Could you check a few things on this model? Use its own coordinates, in mm. Face numbers are marked on the shaded views. A direction names the side the tool comes from. Round coordinates to 2 decimals unless told otherwise and drop trailing zeros. Order: outer loops, then holes, each group sorted by start corner. A loop starts at its lowest first (then second) coordinate and runs counter-clockwise, first axis right, second up.
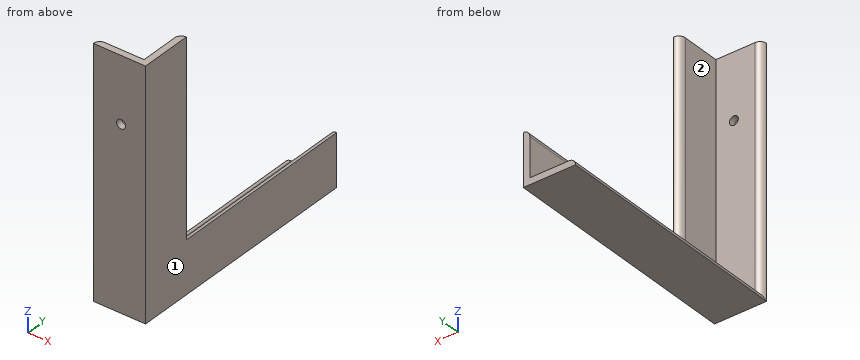
```python
from build123d import *

# Parameters (mm, degrees)
PAD003_DEPTH    = 150
PAD004_DEPTH    = 150
SKETCH012_R     = 2.75
POCKET001_DEPTH = 150.001


with BuildPart() as part:
    # Sketch003 → Pad003 (new body)
    with BuildSketch(Plane.XY):
        with BuildLine():
            Line((0, 32), (0, 0))
            Line((0, 0), (-32, 0))
            ThreePointArc((-28, 4), (-30.828427, 2.828427), (-32, 0))
            Line((-4, 4), (-28, 4))
            Line((-4, 28), (-4, 4))
            ThreePointArc((0, 32), (-2.828427, 30.828427), (-4, 28))
        make_face()
    extrude(amount=PAD003_DEPTH)

    # Sketch004 (on Face3 of Pad003) → Pad004 (new body)
    with BuildSketch(Plane.XZ):
        with BuildLine():
            Line((-32, 0), (0, 0))
            Line((0, 0), (0, 32))
            ThreePointArc((0, 32), (-2.828427, 30.828427), (-4, 28))
            Line((-4, 4), (-4, 28))
            Line((-28, 4), (-4, 4))
            ThreePointArc((-28, 4), (-30.828427, 2.828427), (-32, 0))
        make_face()
    extrude(amount=-PAD004_DEPTH)

    # Sketch012 (on Face9 of Pad004) → Pocket001 (cut, through all)
    with BuildSketch(Plane.XZ):
        with Locations((-15, 110)):
            Circle(SKETCH012_R)
    extrude(amount=-POCKET001_DEPTH, mode=Mode.SUBTRACT)


solid = part.part
```
Q1. For the marked faces 1 and 2, which set-ups out of +Z, -Z, +X, -X, +Y, -Y let a thin tool reach every point of the face, with its end or its side?
Q2. Imagine slicing it at C-C, the plane y = 69.5. Please give me the cut outline in (x, z), then the cut area to 3 significant figures.
Q3. For P1, Ø2, axis at x = -4.5, y = 86.5, coming from the +Z side; P2, Ø7, axis at x = -21.5, z = 76.5, coming from the +Y side; P3, Ø1.5, axis at x = -18.5, y = 111, coming from the +Z side, each with a flat end and sliding along its axis, tell me the tip position at first contact or that it passes through.
Q4. I need wall thicknesses on L1, parallel to Z at x = -15, y = 1.35; L2, parallel to Y at x = -18.5, z = 73. Which ranges of each line are inside material? Lowest first, please.
Q5. Imagine slicing it at B-B, the plane x = -15. Please give me the cut outline in (y, z).
Q6. Imagine slicing it at A-A, the plane z = 110. Please give me the cut outline in (x, y).
Filled in:
1. face 1: +Z, -Z, +X, +Y, -Y
1. face 2: +Z, -X, +Y
2. outline: (-32, 0) - (0, 0) - (0, 32) arc R4 ccw to (-4, 28) - (-4, 4) - (-28, 4) arc R4 ccw to start
2. area: 233 mm2
3. P1: stops at z = 29.94
3. P2: stops at y = 4
3. P3: stops at z = 4
4. L1: z = 0 to 107.25, 112.75 to 150
4. L2: y = 0 to 4
5. outline: (0, 0) - (150, 0) - (150, 4) - (4, 4) - (4, 107.25) - (0, 107.25) - close; (0, 112.75) - (4, 112.75) - (4, 150) - (0, 150) - close
6. outline: (-32, 0) - (-17.75, 0) - (-17.75, 4) - (-28, 4) arc R4 ccw to start; (-12.25, 0) - (0, 0) - (0, 32) arc R4 ccw to (-4, 28) - (-4, 4) - (-12.25, 4) - close
